Can you work these out from the model? Positions are in its coordinate system, mm. Face numbers are marked on the shaded views. Round coordinates to 2 decimals unless told otherwise and drop trailing zeros. Write each loop counter-clockwise with the first axis right and the second up, starting at its lowest first coordinate (ties: lowest second). Pieces come first, ordered by that corner, then holes. Notation, with made-up numbers: (4, -13) - (34, -13) arc R25 ccw to (34, -1) - close; hole circle Ø1 at (78, 1). An arc over 180 degrees is marked (long way). One line per item, written item: value. Start each with the question number.
(1) I want a section at C-C on x = -11. List the corners of the cut face in (y, z) for me.
(2) I'm going to push flat-ended pins straight in: pin 1 Ø3 at (x, y) = (-2, 1.5) entering from +Z; pin 2 Ø0.6 at (x, z) = (9.5, 5) entering from -Y; pin 3 Ø2.5 at (x, z) = (0, -11) entering from -Y. Where does each tip first touch, or does it pass through?
(3) I want a section at A-A on y = 3.75. List the corners of the cut face in (x, z) for me, plus the area to 3 significant figures.
(4) If I drill on L1, parallel to Z at x = 9, y = 4; L2, parallel to Z at x = 0, y = 5.1; L3, parallel to X at y = 2, z = 3.75, over which ranges is the centre line in solid material (lowest first)? Write a range as from..to.
(5) I want a section at D-D on y = 1.75. List the corners of the cut face in (x, z) for me, plus the area to 3 significant figures.
(6) I want a section at B-B on z = -7.5. List the corners of the cut face in (x, y) for me.
(7) Thinking about a two-plate mould opening in X: for the marked faces 1 and 2, which applies, +X half, -X half, draft (parallel to the pull), parting line (faces both ways), or undercut?
from build123d import *
from build123d.topology import SkipClean

# Parameters (mm, degrees)
CUT_EXTRUDE2_DEPTH      = 3.5
CUT_EXTRUDE4_DEPTH      = 2
SKETCH7_R               = 1
CUT_EXTRUDE6_DEPTH      = 7
CUT_EXTRUDE7_DEPTH      = 2.2
CUT_EXTRUDE8_DEPTH      = 12
CUT_EXTRUDE8_DEPTH_BACK = 2


with BuildPart() as part:
    # Sketch1 → Revolve1 (revolve)
    with SkipClean():  # the faces are left unmerged after this step: merging them gives an invalid solid
        with BuildSketch(Plane.XY):
            with BuildLine():
                ThreePointArc((0, 14.4), (-10.182337649, 10.182337649), (-14.4, 0))
                Line((-14.4, 0), (0, 0))
                Line((0, 0), (0, 14.4))
            make_face()
            with BuildLine():
                Line((0, 14.4), (0, 0))
                Line((0, 0), (14.4, 0))
                ThreePointArc((14.4, 0), (10.182337649, 10.182337649), (0, 14.4))
            make_face()
        revolve(axis=Axis((0, -1000, 0), (0, 1, 0)))
    add(part.part.scale(1), mode=Mode.REPLACE)  # the faces are merged on a copy

    # Sketch2 → Cut-Extrude2 (cut)
    with BuildSketch(Plane.XZ):
        Polygon((4.878609775, -8.45), (9.757219549, 0), (4.878609775, 8.45), (-4.878609775, 8.45), (-9.757219549, 0), (-4.878609775, -8.45), align=None)
    extrude(amount=-CUT_EXTRUDE2_DEPTH, mode=Mode.SUBTRACT)

    # Sketch3 → Cut-Extrude4 (cut)
    with BuildSketch(Plane.XZ.offset(-3.5)):
        Polygon((3.723909236, -6.45), (7.447818473, 0), (3.723909236, 6.45), (-3.723909236, 6.45), (-7.447818473, 0), (-3.723909236, -6.45), align=None)
    extrude(amount=-CUT_EXTRUDE4_DEPTH, mode=Mode.SUBTRACT)

    # Sketch4 → Cut-Revolve1 (revolve, cut)
    with BuildSketch(Plane(origin=(0, 0, 0), x_dir=(0, 0, -1), z_dir=(1, 0, 0))):
        with BuildLine():
            Line((-6.45, 5.5), (0, 5.5))
            Line((0, 5.5), (0, 13.5))
            add(Edge.make_bspline(
                [(0, 13.5), (-6.45, 13.5), (-6.45, 5.5)],
                knots=[0, 0, 0, 1.570796327, 1.570796327, 1.570796327], degree=2, weights=[1, 0.707106781, 1]))
        make_face()
    revolve(axis=Axis((0, -1000, 0), (0, 1, 0)), mode=Mode.SUBTRACT)

    # Sketch7 → Cut-Extrude6 (cut)
    with BuildSketch(Plane.XZ):
        with Locations((-9.526279442, 5.5)):
            Circle(SKETCH7_R)
        with Locations((9.526279442, 5.5)):
            Circle(SKETCH7_R)
        with Locations((0, -11)):
            Circle(SKETCH7_R)
    extrude(amount=-CUT_EXTRUDE6_DEPTH, mode=Mode.SUBTRACT)

    # Sketch8 → Cut-Extrude7 (cut)
    with BuildSketch(Plane.XZ):
        Polygon((-8.400446417, 3.55), (-7.274613392, 5.5), (-8.400446417, 7.45), (-10.652112467, 7.45), (-11.777945491, 5.5), (-10.652112467, 3.55), align=None)
        Polygon((7.274613392, 5.5), (8.400446417, 3.55), (10.652112467, 3.55), (11.777945491, 5.5), (10.652112467, 7.45), (8.400446417, 7.45), align=None)
        Polygon((1.125833025, -9.05), (-1.125833025, -9.05), (-2.25166605, -11), (-1.125833025, -12.95), (1.125833025, -12.95), (2.25166605, -11), align=None)
    extrude(amount=-CUT_EXTRUDE7_DEPTH, mode=Mode.SUBTRACT)

    # Sketch9 → Cut-Extrude8 (cut, two sides: drawn at the far end of the back side and taken through both)
    with BuildSketch(Plane.XZ.offset(-3.5).offset(-CUT_EXTRUDE8_DEPTH_BACK)):
        Polygon((4.936344802, -8.55), (9.872689603, 0), (4.936344802, 8.55), (-4.936344802, 8.55), (-9.872689603, 0), (-4.936344802, -8.55), align=None)
    extrude(amount=CUT_EXTRUDE8_DEPTH + CUT_EXTRUDE8_DEPTH_BACK, mode=Mode.SUBTRACT)


solid = part.part
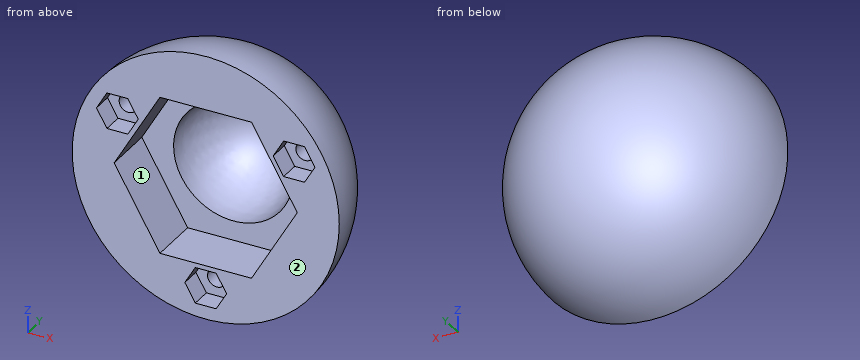
Established:
1. outline: (0, -9.29) arc R9.29 ccw to (0, 9.29) - (0, 6.85) - (2.2, 6.85) - (2.2, 4.15) - (0, 4.15) - close
2. pin 1: z = 14.37
2. pin 2: y = 7
2. pin 3: y = 2.2
3. outline: circle Ø27.81 at (0, 0); hole circle Ø2 at (-9.53, 5.5); hole (-9.87, 0) - (-4.94, -8.55) - (4.94, -8.55) - (9.87, 0) - (4.94, 8.55) - (-4.94, 8.55) - close; hole circle Ø2 at (0, -11); hole circle Ø2 at (9.53, 5.5)
3. area: 345 mm2
4. L1: -10.51..-1.51, 1.51..4.65, 6.35..10.51
4. L2: -13.47..-12, -10..-8.55, 8.55..13.47
4. L3: -13.76..-10.77, -8.28..-7.71, 7.71..8.28, 10.77..13.76
5. outline: circle Ø28.59 at (0, 0); hole (-11.78, 5.5) - (-10.65, 3.55) - (-8.4, 3.55) - (-7.27, 5.5) - (-8.4, 7.45) - (-10.65, 7.45) - close; hole (-9.87, 0) - (-4.94, -8.55) - (4.94, -8.55) - (9.87, 0) - (4.94, 8.55) - (-4.94, 8.55) - close; hole (-2.25, -11) - (-1.13, -12.95) - (1.13, -12.95) - (2.25, -11) - (1.13, -9.05) - (-1.13, -9.05) - close; hole (7.27, 5.5) - (8.4, 3.55) - (10.65, 3.55) - (11.78, 5.5) - (10.65, 7.45) - (8.4, 7.45) - close
5. area: 349 mm2
6. outline: (-12.29, 0) - (-5.54, 0) - (-5.54, 5.5) - (5.54, 5.5) - (5.54, 0) - (12.29, 0) arc R12.29 ccw to start
7. face 1: undercut
7. face 2: draft
